```python
from build123d import *

# Parameters (mm, degrees)
SKETCH1_R           = 50
SKETCH1_R_2         = 27.5
BOSS_EXTRUDE1_DEPTH = 10
FILLET1_R           = 5
SKETCH2_R           = 43
SKETCH2_R_2         = 40
BOSS_EXTRUDE2_DEPTH = 3


with BuildPart() as part:
    # Sketch1 → Boss-Extrude1 (new body)
    with BuildSketch(Plane(origin=(0, 0, 0), x_dir=(1, 0, 0), z_dir=(0, 1, 0))):
        with Locations(Location((0, 0, 0), (0, 0, 270))):
            Circle(SKETCH1_R)
        with Locations(Location((0, 0, 0), (0, 0, 270))):
            Circle(SKETCH1_R_2, mode=Mode.SUBTRACT)
    extrude(amount=BOSS_EXTRUDE1_DEPTH)

    # Fillet1
    fillet1_edges = [part.edges().sort_by_distance(p)[0] for p in [
        (0, 10, -50),
        (0, 10, -27.5),
    ]]
    fillet(fillet1_edges, radius=FILLET1_R)

    # Sketch2 → Boss-Extrude2 (add)
    with BuildSketch(Plane.XZ):
        with Locations(Location((0, 0, 0), (0, 0, 270))):
            Circle(SKETCH2_R)
        with Locations(Location((0, 0, 0), (0, 0, 270))):
            Circle(SKETCH2_R_2, mode=Mode.SUBTRACT)
    extrude(amount=BOSS_EXTRUDE2_DEPTH)


solid = part.part
```
Model file for the job. Use its own axes, mm. A direction names the side the tool comes from. Round coordinates to 2 decimals unless told otherwise and drop trailing zeros. Write each loop counter-clockwise with the first axis right and the second up, starting at its lowest first coordinate (ties: lowest second). Pieces come first, ordered by that corner, then holes. Notation, with made-up numbers: (77, 58) -> (130, 58) arc R28 cw to (130, 86) -> close; hole circle Ø5 at (3, -18). An arc over 180 degrees is marked (long way). Answer as CSV lines item,"result".
1. Pin check, flat tips, straight feed: pin 1 Ø4 at (x, y) = (17, -1) entering from -Z; pin 2 Ø6 at (x, y) = (25.5, 4.5) entering from +Z; pin 3 Ø6 at (y, z) = (0, -17.5) entering from -X. Stop position of each tip, or through.
Resolved:
pin 1,"z = -47.61"
pin 2,"z = 44.65"
pin 3,"x = -47.85"
2. Slice it at A-A, the plane x = 0. List the corners of the cut face in (y, z), plus the area to 3 significant figures.
Resolved:
outline,"(-3, -43) -> (0, -43) -> (0, -50) -> (5, -50) arc R5 ccw to (10, -45) -> (10, -32.5) arc R5 ccw to (5, -27.5) -> (0, -27.5) -> (0, -40) -> (-3, -40) -> close; (-3, 40) -> (0, 40) -> (0, 27.5) -> (5, 27.5) arc R5 ccw to (10, 32.5) -> (10, 45) arc R5 ccw to (5, 50) -> (0, 50) -> (0, 43) -> (-3, 43) -> close"
area,"447 mm²"
3. Mould opens along X. For faces 1 (the face through (15.02, 2.46, 47.69)), 2 (the face through (-39.05, -1.48, 8.67)), 3 (the face through (-30, 10, 13)) say: +X half, -X half, draft (parallel to the pull), parting line (faces both ways), or undercut.
Resolved:
face 1,"parting line"
face 2,"undercut"
face 3,"draft"
4. Tool access for faces 4 (the face through (-26.1, 0, -9.4)), 5 (the face through (-24.397, 2.465, 12.69)): list every direction of +Z, -Z, +X, -X, +Y, -Y with a clear straight run to the whole face (end or side of a thin tool).
Resolved:
face 4,"-Y"
face 5,"+Y, -Y"
5. Slice it at B-B, the plane z = 0. List the corners of the cut face in (x, y).
Resolved:
outline,"(-50, 0) -> (-43, 0) -> (-43, -3) -> (-40, -3) -> (-40, 0) -> (-27.5, 0) -> (-27.5, 5) arc R5 ccw to (-32.5, 10) -> (-45, 10) arc R5 ccw to (-50, 5) -> close; (27.5, 0) -> (40, 0) -> (40, -3) -> (43, -3) -> (43, 0) -> (50, 0) -> (50, 5) arc R5 ccw to (45, 10) -> (32.5, 10) arc R5 ccw to (27.5, 5) -> close"
6. Drill centre lines: line 1 (X direction, y = 1.7, z = 0); line 2 (X direction, y = -2.3, z = 0); line 3 (Y direction, x = -9.5, z = 31). Where is each one in solid material? Low to high.
Resolved:
line 1,"-50 to -27.5, 27.5 to 50"
line 2,"-43 to -40, 40 to 43"
line 3,"0 to 10"
7. Slice it at C-C, the plane y = 6.5. List the corners of the cut face in (x, z), plus the area to 3 significant figures.
Resolved:
outline,"circle Ø99.54 at (0, 0); hole circle Ø55.46 at (0, 0)"
area,"5,370 mm²"
